Build history of the part. All positions in model axes, mm. A direction names the side the tool comes from. Coordinates: 2 decimals unless noted, no trailing zeros. Loops run counter-clockwise (first coordinate to the right, second up) from the corner with the lowest first, then second, coordinate; pieces in that order, holes last. Notation, with made-up numbers: (-29.75, 56.5) - (3.25, 56.5) arc R21 cw to (3.25, 91.5) - close; hole circle Ø3 at (-26, -15). An arc over 180 degrees is marked (long way). One line per item, written item: value.
Autodesk Inventor part; units mm, degrees
ref_plane "YZ Plane" through (0, 0, 0) normal (1, 0, 0) x (0, 1, 0)
ref_plane "XZ Plane" through (0, 0, 0) normal (0, 1, 0) x (-1, 0, 0)
ref_plane "XY Plane" through (0, 0, 0) normal (0, 0, 1) x (1, 0, 0)
sketch "Sketch1" plane through (0, 0, 0) normal (0, 0, 1) x (1, 0, 0)
  line L0 (0, 0) -> (25.4, 0)
  line L1 (25.4, 0) -> (25.4, 25.4)
  line L2 (25.4, 25.4) -> (0, 25.4)
  line L3 (0, 25.4) -> (0, 0)
  line L4 (1.5875, 23.8125) -> (23.8125, 23.8125)
  line L5 (23.8125, 23.8125) -> (23.8125, 1.5875)
  line L6 (23.8125, 1.5875) -> (1.5875, 1.5875)
  line L7 (1.5875, 1.5875) -> (1.5875, 23.8125)
  dimension "d0" = 25.4
  dimension "d1" = 25.4
  dimension "d2" = 1.5875
extrude "Extrusion1" add sketch "Sketch1" against normal blind 152.4
sketch "Sketch2" plane through (0, 0, 0) normal (0, -1, 0) x (1, 0, 0)
  line L0 (0, -152.4) -> (25.4, -152.4)
  line L1 (0, 0) -> (25.4, 0)
  point P0 (12.7, -12.7)
  point P1 (12.7, -139.7)
  point P2 (12.7, -114.3)
  point P3 (12.7, -88.9)
  point P4 (12.7, -152.4)
  dimension "d5" = 25.4
  dimension "d6" = 25.4
  dimension "d7" = 12.7
  dimension "d8" = 12.7
hole "Hole1" at (12.7, 0, -12.7) at (12.7, 0, -139.7) at (12.7, 0, -114.3) at (12.7, 0, -88.9) direction (0, 1, 0) diameter 6.35 depth 25.4 tip angle 118
sketch "Sketch3" plane through (0, 0, 0) normal (-1, 0, 0) x (0, 0, 1)
  line L0 (-152.4, 25.4) -> (-152.4, 0)
  point P0 (-139.7, 12.7)
  point P1 (-101.6, 12.7)
  dimension "d25" = 12.7
  dimension "d27" = 38.1
hole "Hole2" at (0, 12.7, -139.7) at (0, 12.7, -101.6) direction (1, 0, 0) diameter 6.35 depth 25.4 tip angle 118
properties part number "1tube_6"
Item 1: Drop a flat-ended pin along its axis: P1, Ø5, axis at y = 12.7, z = -139.7, coming from the +X side. Give the stop position or say it passes through.
Check result:
P1: passes through
Item 2: Tool access for faces 1 (the face through (1.588, 13, -75)), 2 (the face through (0.8, 13.92, -136.77)): list every direction of +Z, -Z, +X, -X, +Y, -Y with a clear straight run to the whole face (end or side of a thin tool).
Check result:
face 1: +Z, -Z
face 2: +X, -X
Item 3: Probe probe 1 along Z at (x, y) = (12.7, 1) (3 decimals); probe 2 along Y at (x, z) = (12.5, -40); probe 3 along Y at (x, z) = (24.7, -139.7) (3 decimals). List the from-to ranges inside material, lowest first. Write a range as from..to.
Check result:
probe 1: z = -152.4..-142.875, -136.525..-117.475, -111.125..-92.075, -85.725..-15.875, -9.525..0
probe 2: y = 0..1.59, 23.81..25.4
probe 3: y = 0..9.525, 15.875..25.4
Item 4: Cut at B-B, the plane x = 6.5. Write the cut outline in (y, z), then the cut area to 3 significant figures.
Check result:
outline: (0, -152.4) - (1.59, -152.4) - (1.59, 0) - (0, 0) - close; (23.81, -152.4) - (25.4, -152.4) - (25.4, 0) - (23.81, 0) - close
area: 484 mm^2
Item 5: Pull direction Z, two halves, no side cores. Call faces 3 (the face through (1, 13, 0)), 4 (the face through (23.812, 13, -75)), 5 (the face through (1, 13, -152.4)), 6 (the face through (24.62, 14.63, -104.12)): released by +Z, released by -Z, zero draft, split by the parting line, or undercut.
Check result:
face 3: released by +Z
face 4: zero draft
face 5: released by -Z
face 6: undercut
Item 6: Cut at A-A, the plane z = -101.6. Write the cut outline in (x, y) (1 decimal).
Check result:
outline: (0, 0) - (25.4, 0) - (25.4, 9.5) - (23.8, 9.5) - (23.8, 1.6) - (1.6, 1.6) - (1.6, 9.5) - (0, 9.5) - close; (0, 15.9) - (1.6, 15.9) - (1.6, 23.8) - (23.8, 23.8) - (23.8, 15.9) - (25.4, 15.9) - (25.4, 25.4) - (0, 25.4) - close
Item 7: Cut at D-D, the plane z = -139.7. Write the cut outline in (x, y) (1 decimal), then the cut area to 3 significant figures.
Check result:
outline: (0, 0) - (9.5, 0) - (9.5, 1.6) - (1.6, 1.6) - (1.6, 9.5) - (0, 9.5) - close; (0, 15.9) - (1.6, 15.9) - (1.6, 23.8) - (9.5, 23.8) - (9.5, 25.4) - (0, 25.4) - close; (15.9, 0) - (25.4, 0) - (25.4, 9.5) - (23.8, 9.5) - (23.8, 1.6) - (15.9, 1.6) - close; (15.9, 23.8) - (23.8, 23.8) - (23.8, 15.9) - (25.4, 15.9) - (25.4, 25.4) - (15.9, 25.4) - close
area: 111 mm^2
